```python
from build123d import *

# Parameters (mm, degrees)
SKETCH1_W                                          = 44
SKETCH1_H                                          = 15.3
SKETCH1_R                                          = 1
BOSS_EXTRUDE1_DEPTH                                = 2.5
CBORE_FOR_M2_5_PAN_HEAD_MACHINE_SCREW1_D           = 2.7
CBORE_FOR_M2_5_PAN_HEAD_MACHINE_SCREW1_CBORE_D     = 6
CBORE_FOR_M2_5_PAN_HEAD_MACHINE_SCREW1_CBORE_DEPTH = 1
CUT_EXTRUDE1_DEPTH                                 = 1
FILLET1_R                                          = 1
FILLET2_R                                          = 0.25


with BuildPart() as part:
    # Sketch1 → Boss-Extrude1 (new body)
    with BuildSketch(Plane(origin=(0, 0, 0), x_dir=(0, 0, -1), z_dir=(1, 0, 0))):
        Rectangle(SKETCH1_W, SKETCH1_H)
        Circle(SKETCH1_R, mode=Mode.SUBTRACT)
    extrude(amount=BOSS_EXTRUDE1_DEPTH)

    # CBORE for M2.5 Pan Head Machine Screw1 (through all)
    with Locations(Plane(origin=(2.5, 0, 0), x_dir=(0, 0, -1), z_dir=(1, 0, 0))):
        with Locations((-18.125, 5), (19.5, 5)):
            CounterBoreHole(CBORE_FOR_M2_5_PAN_HEAD_MACHINE_SCREW1_D / 2, CBORE_FOR_M2_5_PAN_HEAD_MACHINE_SCREW1_CBORE_D / 2, CBORE_FOR_M2_5_PAN_HEAD_MACHINE_SCREW1_CBORE_DEPTH)

    # Sketch5 → Cut-Extrude1 (cut)
    with BuildSketch(Plane(origin=(2.5, 0, 0), x_dir=(0, 0, -1), z_dir=(1, 0, 0))):
        with BuildLine():
            ThreePointArc((22, 6.658312395), (21.515075982, 7.222491571), (20.906236111, 7.65))
            Line((20.906236111, 7.65), (22, 7.65))
            Line((22, 7.65), (22, 6.658312395))
        make_face()
    extrude(amount=-CUT_EXTRUDE1_DEPTH, mode=Mode.SUBTRACT)

    # Fillet1
    fillet1_edges = [part.edges().sort_by_distance(p)[0] for p in [
        (2, 3.341687605, -22),
        (2, 7.65, -18.093763889),
        (2, 7.65, 16.718763889),
        (0.75, 7.65, -22),
        (1.25, -7.65, -22),
        (1.25, -7.65, 22),
        (1.25, 7.65, 22),
    ]]
    fillet(fillet1_edges, radius=FILLET1_R)

    # Fillet2
    fillet2_edges = [part.edges().sort_by_distance(p)[0] for p in [
        (2, 7.65, 19.531236111),
    ]]
    fillet(fillet2_edges, radius=FILLET2_R)


solid = part.part
```
Verification items for the finished model (mm, model axes). A direction names the side the tool comes from. Round coordinates to 2 decimals unless told otherwise and drop trailing zeros. Write each loop counter-clockwise with the first axis right and the second up, starting at its lowest first coordinate (ties: lowest second). Pieces come first, ordered by that corner, then holes. Notation, with made-up numbers: (-32.75, -32) -> (20.25, -32) arc R18 cw to (20.25, -5) -> close; hole circle Ø5 at (44, -38). An arc over 180 degrees is marked (long way). Write each question's results on one line, items separated by ' | '. Start each with the question number.
1. Depth check by flat-ended pin: P1, Ø2.5, axis at y = 5, z = 18.125, coming from the -X side; P2, Ø3, axis at y = 5.5, z = -20, coming from the +X side. Enter the tip coordinate at first touch or a pass-through.
2. Cross-section at C-C (y = 5). Enter the section's corners in (x, z) (3 decimals), then the cut area to 3 significant figures.
3. Cross-section at B-B (y = 0). Enter the section's corners in (x, z).
4. Cross-section at D-D (x = 0.8). Enter the section's corners in (y, z) (3 decimals).
5. Set-up check for faces 4 (the cylindrical face through (2.007, 7.18, -16.704)), 5 (the cylindrical face through (2.007, 2.129, -21.548)), 6 (the cylindrical face through (2.01, 2.08, 18.82)): record each of +Z, -Z, +X, -X, +Y, -Y from which the full face is reachable in a straight line by a thin tool's end or side.
6. Cross-section at A-A (z = 0). Enter the section's corners in (x, y), then the cut area to 4 significant figures.
7. Draft check along X on faces 1 (the flat face through (0, -2, 0)), 2 (the cylindrical face through (0.74, 5.406, -18.212)), 3 (the flat face through (1.5, 6, -18)). Enter one of: +X half, -X half, draft (parallel to the pull), parting line (faces both ways), or undercut.
8. Material ranges on probe 1 along Y at (x, z) = (0.55, -19.5); probe 2 along Z at (x, y) = (0.25, 0.5); probe 3 along X at (y, z) = (6, 16.5), recorded low to high. Write a range as from..to.
Solutions:
1) P1: passes through | P2: stops at x = 1.5
2) outline: (0, -22) -> (1.5, -22) -> (1.5, -20.85) -> (0, -20.85) -> close; (0, -18.15) -> (1.5, -18.15) -> (1.5, -16.5) -> (2.5, -16.5) -> (2.5, 15.125) -> (1.5, 15.125) -> (1.5, 16.775) -> (0, 16.775) -> close; (0, 19.475) -> (1.5, 19.475) -> (1.5, 21.125) -> (2.5, 21.125) -> (2.5, 22) -> (0, 22) -> close | area: 90.4 mm2
3) outline: (0, -22) -> (2.5, -22) -> (2.5, -1) -> (0, -1) -> close; (0, 1) -> (2.5, 1) -> (2.5, 22) -> (0, 22) -> close
4) outline: (-7.65, -21) arc R1 ccw to (-6.65, -22) -> (6.65, -22) arc R1 ccw to (7.65, -21) -> (7.65, 21) arc R1 ccw to (6.65, 22) -> (-6.65, 22) arc R1 ccw to (-7.65, 21) -> close; hole circle Ø2 at (0, 0); hole circle Ø2.7 at (5, -19.5); hole circle Ø2.7 at (5, 18.125)
5) face 4: -Z, +X | face 5: +X, +Y | face 6: +X
6) outline: (0, -7.65) -> (2.5, -7.65) -> (2.5, -1) -> (0, -1) -> close; (0, 1) -> (2.5, 1) -> (2.5, 7.65) -> (0, 7.65) -> close | area: 33.25 mm2
7) face 1: -X half | face 2: draft | face 3: +X half
8) probe 1: y = -7.65..3.65, 6.35..7.65 | probe 2: z = -22..-0.87, 0.87..22 | probe 3: x = 0..1.5
